```python
from build123d import *

# Parameters (mm, degrees)
F1_DEPTH       = 18
F3_DEPTH       = 13.9
F5_DEPTH       = 12
F7_D           = 6.6
F7_CBORE_D     = 11.25
F7_CBORE_DEPTH = 6
F8_R           = 3


with BuildPart() as f1:
    # F0 (on Front) → F1 (new body)
    with BuildSketch(Plane.XZ):
        Polygon((0, 12), (0, 0), (48, 0), (48, 12), (30.25, 24), (17.75, 24), align=None)
    extrude(amount=F1_DEPTH)

    # F2 (on face) → F3 (cut)
    with BuildSketch(Plane.XZ.offset(18)):
        with BuildLine():
            ThreePointArc((20.5358983849, 24), (22.9647238196, 18.1362966948), (28, 22))
            ThreePointArc((28, 22), (27.8637033052, 23.0352761804), (27.4641016151, 24))
            Line((27.4641016151, 24), (20.5358983849, 24))
        make_face()
    extrude(amount=-F3_DEPTH, mode=Mode.SUBTRACT)

    # F4 (on face) → F5 (cut)
    with BuildSketch(Plane.XY.offset(24)):
        with BuildLine():
            Line((8.5, -3.375), (0, -3.375))
            Line((0, -3.375), (0, -18))
            Line((0, -18), (14.125, -18))
            Line((14.125, -18), (14.125, -9))
            ThreePointArc((14.125, -9), (12.4774756442, -5.0225243558), (8.5, -3.375))
        make_face()
        with BuildLine():
            ThreePointArc((39.5, -3.375), (35.5225243558, -5.0225243558), (33.875, -9))
            Line((33.875, -9), (33.875, -18))
            Line((33.875, -18), (48, -18))
            Line((48, -18), (48, -3.375))
            Line((48, -3.375), (39.5, -3.375))
        make_face()
    extrude(amount=-F5_DEPTH, mode=Mode.SUBTRACT)

    # F7 (through all)
    with Locations(Plane.XY.offset(12)):
        with Locations((8.5, -9), (39.5, -9)):
            CounterBoreHole(F7_D / 2, F7_CBORE_D / 2, F7_CBORE_DEPTH)

    # F8
    f8_edges = [f1.edges().sort_by_distance(p)[0] for p in [
        (0, 0, 6),
        (0, -18, 6),
        (48, -18, 6),
        (48, 0, 6),
    ]]
    fillet(f8_edges, radius=F8_R)


solid = f1.part
```
Design review of the part built by this model. Coordinates are the model's own, in mm. A direction names the side the tool comes from. Give positions to 0.01 mm unless a question says otherwise; leave off trailing zeros. Loops run counter-clockwise (first coordinate to the right, second up) from the corner with the lowest first, then second, coordinate; pieces in that order, holes last. Notation, with made-up numbers: (22.25, 81.5) -> (72.25, 81.5) arc R17 cw to (72.25, 108.5) -> close; hole circle Ø9 at (49.25, -27.5). An arc over 180 degrees is marked (long way). One line per item, written item: value.
Q1. Machinability: for faces 1 (the flat face through (44, -14, 12)), 2 (the flat face through (12.94, -4.87, 20.75)), 3 (the flat face through (0, -9, 6)), 4 (the cylindrical face through (35.35, -5.2, 10.43)), 5 (the flat face through (6, -3.375, 14)), which of the approach directions +Z, -Z, +X, -X, +Y, -Y give a long, thin tool a straight path to every point of the face, cutting with its end or side? Answer none if there is none.
Numbers:
face 1: +Z, +X, -Y
face 2: +Z, -X, +Y, -Y
face 3: +Z, -Z, -X, +Y, -Y
face 4: +Z
face 5: +Z, -X, -Y
Q2. For pin 1 Ø9 at (x, y) = (8.5, -8.5) entering from +Z; pin 2 Ø1.7 at (x, z) = (44, 13.5) entering from -Y (3 decimals); pin 3 Ø3 at (y, z) = (-6, 18.5) entering from -X (3 decimals), all flat-tipped, find the tip position at first contact; note any pin that passes through.
Numbers:
pin 1: stops at z = 6
pin 2: stops at y = -3.375
pin 3: stops at x = 11.875
Q3. For L1, parallel to X at y = -9, z = 11.5 (3 decimals); L2, parallel to X at y = -10, z = 5.5; L3, parallel to Y at x = 39.5, z = 4.5, list the stretches that pass through material, from the lowest coordinate up.
Numbers:
L1: x = 0 to 2.875, 14.125 to 33.875, 45.125 to 48
L2: x = 0 to 5.36, 11.64 to 36.36, 42.64 to 48
L3: y = -18 to -12.3, -5.7 to 0
Q4. We need section C-C on x = 24. Give the boundary of the cut face in (y, z).
Numbers:
outline: (-18, 0) -> (0, 0) -> (0, 24) -> (-4.1, 24) -> (-4.1, 18) -> (-18, 18) -> close
Q5. Draft analysis for pull direction Y (two halves, no side actions). For faces 6 (the flat face through (12, -9, 6)), 7 (the flat face through (48, -9, 6)), 8 (the cylindrical face through (0.86, -17.1, 5.92)), state which applies: pulls with the +Y half, pulls with the -Y half, needs draft (parallel to the pull), parting line crosses it, or undercut.
Numbers:
face 6: undercut
face 7: needs draft
face 8: pulls with the -Y half
Q6. We need section B-B on y = -10. Give the boundary of the cut face in (x, z) (3 decimals), and give its area (3 significant figures).
Numbers:
outline: (0, 0) -> (5.355, 0) -> (5.355, 6) -> (2.965, 6) -> (2.965, 12) -> (0, 12) -> close; (11.645, 0) -> (36.355, 0) -> (36.355, 6) -> (33.965, 6) -> (33.965, 12) -> (33.875, 12) -> (33.875, 21.549) -> (30.25, 24) -> (27.464, 24) arc R4 cw (long way) to (20.536, 24) -> (17.75, 24) -> (14.125, 21.549) -> (14.125, 12) -> (14.035, 12) -> (14.035, 6) -> (11.645, 6) -> close; (42.645, 0) -> (48, 0) -> (48, 12) -> (45.035, 12) -> (45.035, 6) -> (42.645, 6) -> close
area: 555 mm^2
Q7. We need section A-A on z = 10.25. Give the boundary of the cut face in (x, y) (3 decimals), and give its area (3 significant figures).
Numbers:
outline: (0, -15) arc R3 ccw to (3, -18) -> (45, -18) arc R3 ccw to (48, -15) -> (48, -3) arc R3 ccw to (45, 0) -> (3, 0) arc R3 ccw to (0, -3) -> close; hole circle Ø11.25 at (8.5, -9); hole circle Ø11.25 at (39.5, -9)
area: 657 mm^2
